Geometry: final body of the model. Coordinates: model frame, mm. A direction names the side the tool comes from. Coordinates: 2 decimals unless noted, no trailing zeros. Loops run counter-clockwise (first coordinate to the right, second up) from the corner with the lowest first, then second, coordinate; pieces in that order, holes last. Notation, with made-up numbers: M 9,-14.5 L 14,-14.5 A17 ccw 14,-1.5 Z; hole C 73,22.25 d2. An arc over 180 degrees is marked long. Write item = value, one per line. Start each with the question number.
```python
from build123d import *

# Parameters (mm, degrees)
BOSS_EXTRUDE1_DEPTH      = 7
BOSS_EXTRUDE2_DEPTH      = 3
BOSS_EXTRUDE2_DEPTH_BACK = 10
SKETCH2_W                = 20
SKETCH2_H                = 8
FILLET1_R                = 6
FILLET2_R                = 3
F_3_0_3_DIAMETER_HOLE1_D = 3


with BuildPart() as part:
    # Sketch1 → Boss-Extrude1 (new body)
    with BuildSketch(Plane(origin=(0, 0, 0), x_dir=(1, 0, 0), z_dir=(0, 1, 0))):
        Polygon((50, 0), (50, 8), (30, 8), (0, 23), (-40, 2), (-40, 0), (-30, 0), (0, 15), (30, 0), align=None)
    extrude(amount=BOSS_EXTRUDE1_DEPTH)

    # Sketch2 → Boss-Extrude2 (add, two sides: drawn at the far end of the back side and taken through both)
    with BuildSketch(Plane(origin=(0, 7, 0), x_dir=(1, 0, 0), z_dir=(0, 1, 0)).offset(-BOSS_EXTRUDE2_DEPTH_BACK)):
        with Locations((40, 4)):
            Rectangle(SKETCH2_W, SKETCH2_H)
    extrude(amount=BOSS_EXTRUDE2_DEPTH + BOSS_EXTRUDE2_DEPTH_BACK)

    # Fillet1
    fillet1_edges = [part.edges().sort_by_distance(p)[0] for p in [
        (50, -3, -4),
        (50, 10, -4),
    ]]
    fillet(fillet1_edges, radius=FILLET1_R)

    # Fillet2
    fillet2_edges = [part.edges().sort_by_distance(p)[0] for p in [
        (30, -3, -4),
        (30, 10, -4),
    ]]
    fillet(fillet2_edges, radius=FILLET2_R - 0.0001)  # a hair under: the kernel refuses the full size

    # Ø3.0 (3) Diameter Hole1 (through all)
    with Locations(Plane(origin=(0, 0, -8), x_dir=(-1, 0, 0), z_dir=(0, 0, -1))):
        with Locations((-44, 3.5), (-34.5, 3.5)):
            Hole(F_3_0_3_DIAMETER_HOLE1_D / 2)


solid = part.part
```
Item 1: Section query B-B (z = -5). Count the separate pieces of the cut face and the enclosed holes in it, plus the area to 3 significant figures.
Item 2: Section query A-A (x = 34.5). Return the cut outline in (y, z), plus the area to 3 significant figures.
Item 3: Reachability of faces 1 (the flat face through (-3, 7, -14)), 2 (the flat face through (-3, 0, -14)), 3 (the flat face through (14.8, 3.5, -7.6)) from +Z, -Z, +X, -X, +Y, -Y: full face, straight path, thin tool, end or side. Return the list, or none.
Item 4: Section query C-C (x = 19). Return the cut outline in (y, z).
Item 5: Section query D-D (z = -17.5). Return the cut outline in (x, y), plus the area to 3 significant figures.
Item 6: Line query: line 1 (Y direction, x = 34.5, z = -4.5); line 2 (X direction, y = 5.25, z = -13.25); line 3 (Z direction, x = 31, y = -0.5). Output: solid intervals per line, ascending. Write a range as from..to.
Item 7: First-contact query: pin 1 (2.5 mm diameter, centred on x = 44, y = 3.5, fed in from -Z); pin 2 (4 mm diameter, centred on x = 34.5, y = 3.5, fed in from -Z); pin 3 (1 mm diameter, centred on x = -16, z = -15, fed in from +Y); pin 4 (1 mm diameter, centred on x = -8.5, z = -17, fed in from -Y). Flat tips, straight axial feed; report the tip coordinate or a pass-through.
Verdict:
q1.separate_pieces = 2
q1.enclosed_holes = 2
q1.area = 397 mm2
q2.outline = M -3,-8 L 2,-8 L 2,0 L -3,0 Z; M 5,-8 L 10,-8 L 10,0 L 5,0 Z
q2.area = 80.0 mm2
q3.face_1 = +Z, -Z, -X, +Y
q3.face_2 = +Z, -Z, -X, -Y
q3.face_3 = +Z, +Y, -Y
q4.outline = M 0,-13.5 L 7,-13.5 L 7,-5.5 L 0,-5.5 Z
q5.outline = M -10.48,0 L 11,0 L 11,7 L -10.48,7 Z
q5.area = 150 mm2
q6.line_1 = -3..2, 5..10
q6.line_2 = -18.57..-3.5, 3.5..19.5
q6.line_3 = -8..0
q7.pin_1 = through
q7.pin_2 = -8
q7.pin_3 = 7
q7.pin_4 = 0
